Build history of the part. All positions in model axes, mm. Coordinates: 2 decimals unless noted, no trailing zeros. Order: outer loops, then holes, each group sorted by start corner. A loop starts at its lowest first (then second) coordinate and runs counter-clockwise, first axis right, second up. Notation, with made-up numbers: M 25.5,-11 L 39.5,-11 A29 cw 39.5,20 Z; hole C 66.25,-6.75 d4. An arc over 180 degrees is marked long. Write item = value, one per line. Start each with the question number.
Q1. Pin check, flat tips, straight feed: P1, Ø6, axis at x = 42.5, z = 19, coming from the +Y side; P2, Ø1.8, axis at y = -10, z = 21, coming from the -X side; P3, Ø3.5, axis at y = -10, z = 20, coming from the +X side. Stop position of each tip, or through.
Q2. Drill centre line: probe 1 along Z at (x, y) = (-144.75, -10). Where is it in solid material? Low to high.
Q3. Band-saw the part on A-A on z = 20. Write the cut outline in (x, y).
```python
from build123d import *

# Parameters (mm, degrees)
F0_W     = 324
F0_H     = 40
F1_DEPTH = 20
F2_R     = 3
F4_DEPTH = 12
F3_R     = 3
F5_DEPTH = 12


with BuildPart() as f1:
    # F0 (on Front) → F1 (new body)
    with BuildSketch(Plane.XZ):
        with Locations((7.898747, 20)):
            Rectangle(F0_W, F0_H)
    extrude(amount=F1_DEPTH)

    # F2 (on face) → F4 (cut)
    with BuildSketch(Plane.YZ.offset(169.898747)):
        with Locations((-10, 20)):
            Circle(F2_R)
    extrude(amount=-F4_DEPTH, mode=Mode.SUBTRACT)

    # F3 (on face) → F5 (cut)
    with BuildSketch(Plane(origin=(-154.101253, 0, 0), x_dir=(0, -1, 0), z_dir=(-1, 0, 0))):
        with Locations((10, 20)):
            Circle(F3_R)
    extrude(amount=-F5_DEPTH, mode=Mode.SUBTRACT)


solid = f1.part
```
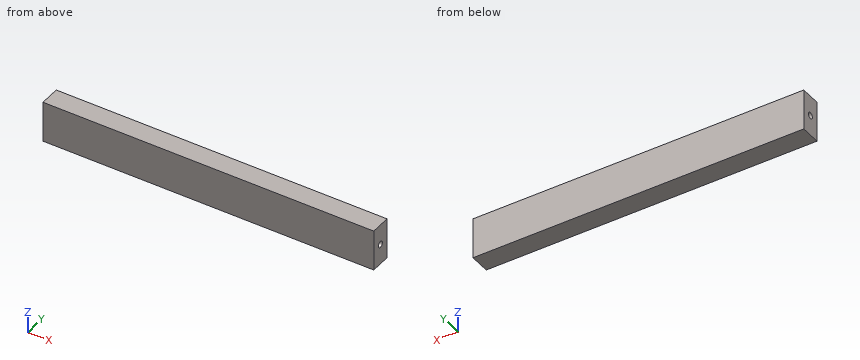
Recorded:
q1.P1 = 0
q1.P2 = -142.1
q1.P3 = 157.9
q2.probe_1 = 0 to 17, 23 to 40
q3.outline = M -154.1,-20 L 169.9,-20 L 169.9,-13 L 157.9,-13 L 157.9,-7 L 169.9,-7 L 169.9,0 L -154.1,0 L -154.1,-7 L -142.1,-7 L -142.1,-13 L -154.1,-13 Z
